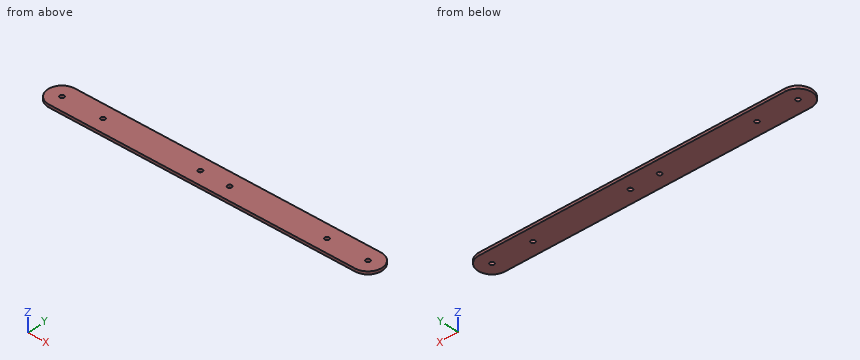
from build123d import *

# Parameters (mm, degrees)
SKETCH_1_R      = 1.55
EXTRUDE_1_DEPTH = 2


with BuildPart() as part:
    # 草图1 → 凸台-拉伸1 (new body)
    with BuildSketch(Plane.XY):
        with BuildLine():
            Line((-110, 10), (110, 10))
            ThreePointArc((110, 10), (120, 0), (110, -10))
            Line((110, -10), (-110, -10))
            ThreePointArc((-110, -10), (-120, 0), (-110, 10))
        make_face()
        with Locations((10.5, 0)):
            Circle(SKETCH_1_R, mode=Mode.SUBTRACT)
        with Locations((80.5, 0)):
            Circle(SKETCH_1_R, mode=Mode.SUBTRACT)
        with Locations(Location((-80.5, 0, 0), (0, 0, 180))):
            Circle(SKETCH_1_R, mode=Mode.SUBTRACT)
        with Locations(Location((-10.5, 0, 0), (0, 0, 180))):
            Circle(SKETCH_1_R, mode=Mode.SUBTRACT)
        with Locations((-110, 0)):
            Circle(SKETCH_1_R, mode=Mode.SUBTRACT)
        with Locations(Location((110, 0, 0), (0, 0, 180))):
            Circle(SKETCH_1_R, mode=Mode.SUBTRACT)
    extrude(amount=EXTRUDE_1_DEPTH)


solid = part.part
Source: CAD feature listing. Evaluate the final solid. Frame: model axes, mm. Coordinates: 2 decimals unless noted, no trailing zeros. Write each loop counter-clockwise with the first axis right and the second up, starting at its lowest first coordinate (ties: lowest second). Pieces come first, ordered by that corner, then holes. Notation, with made-up numbers: M -20.5,-40 L 22.5,-40 A8 ccw 22.5,-33 Z; hole C 81.25,52.5 d9. An arc over 180 degrees is marked long. Use a Markdown table: item, result.
1) Section A-A, the plane z = 1.55. Output: boundary loops of the cut face in (x, y).
Conclusion:
| item | result |
|---|---|
| outline | M -110,-10 L 110,-10 A10 ccw 110,10 L -110,10 A10 ccw Z; hole C -110,0 d3.1; hole C -80.5,0 d3.1; hole C -10.5,0 d3.1; hole C 10.5,0 d3.1; hole C 80.5,0 d3.1; hole C 110,0 d3.1 |
2) First-contact query: pin 1 Ø2.5 at (x, y) = (10.5, 0) entering from -Z; pin 2 Ø1 at (y, z) = (-3, 0.5) entering from +X. Flat tips, straight axial feed; report the tip coordinate or a pass-through.
Conclusion:
| item | result |
|---|---|
| pin 1 | passes through |
| pin 2 | stops at x = 119.68 |
3) Section B-B, the plane y = 7.5. Output: boundary loops of the cut face in (x, z).
Conclusion:
| item | result |
|---|---|
| outline | M -116.61,0 L 116.61,0 L 116.61,2 L -116.61,2 Z |
4) Ray query, L1, parallel to Y at x = 80.5, z = 0.8; L2, parallel to Y at x = 79.5, z = 1.2; L3, parallel to X at y = 9, z = 1.6. Return the intervals inside material, ascending.
Conclusion:
| item | result |
|---|---|
| L1 | y = -10 to -1.55, 1.55 to 10 |
| L2 | y = -10 to -1.18, 1.18 to 10 |
| L3 | x = -114.36 to 114.36 |
